Can you work these out from the model? Positions are in its coordinate system, mm. A direction names the side the tool comes from. Give positions to 0.01 mm unless a question says otherwise; leave off trailing zeros. Order: outer loops, then holes, each group sorted by start corner. A loop starts at its lowest first (then second) coordinate and runs counter-clockwise, first axis right, second up. Notation, with made-up numbers: M -32.75,54.5 L -19.75,54.5 A21 cw -19.75,83.5 Z; hole C -35,55.25 d3. An arc over 180 degrees is marked long. Write each question's results on one line, items separated by ' | '.
from build123d import *

# Parameters (mm, degrees)
F0_R     = 30
F0_R_2   = 20
F0_R_3   = 3.5
F1_DEPTH = 35
F2_DEPTH = 45
F3_DEPTH = 65
F6_DEPTH = 10
F7_R     = 3.5


with BuildPart() as f1:
    # F0 (on Top) → F1 (new body)
    with BuildSketch(Plane.XY):
        Circle(F0_R)
        Circle(F0_R_2, mode=Mode.SUBTRACT)
        Circle(F0_R_2)
        Circle(F0_R_3, mode=Mode.SUBTRACT)
    extrude(amount=-F1_DEPTH)

    # F0 (on Top) → F2 (join)
    with BuildSketch(Plane.XY):
        Circle(F0_R_2)
        Circle(F0_R_3, mode=Mode.SUBTRACT)
    extrude(amount=F2_DEPTH)

    # F0 (on Top) → F3 (join)
    with BuildSketch(Plane.XY):
        Circle(F0_R_3)
    extrude(amount=F3_DEPTH)

    # F5 (on offset) → F6 (join)
    with BuildSketch(Plane.XY.offset(65)):
        with BuildLine():
            Line((0, 3.582485), (0, 15))
            ThreePointArc((0, 15), (-10.606602, 10.606602), (-15, 0))
            Line((-15, 0), (-1.836112, 0))
            Line((-1.836112, 0), (-0.225955, 0))
            Line((-0.225955, 0), (0, -0.090901))
            Line((0, -0.090901), (0, -1.836112))
            Line((0, -1.836112), (0, -15))
            ThreePointArc((0, -15), (10.606602, -10.606602), (15, 0))
            Line((15, 0), (1.836112, 0))
            Line((1.836112, 0), (0.280118, 0))
            Line((0.280118, 0), (0, 0.357013))
            Line((0, 0.357013), (0, 3.582485))
        make_face()
    extrude(amount=F6_DEPTH)

    # F7
    f7_edges = [f1.edges().sort_by_distance(p)[0] for p in [
        (-20, 0, 45),
        (-30, 0, 0),
    ]]
    fillet(f7_edges, radius=F7_R)


solid = f1.part
(1) For faces 1 (the face through (7, -7, 65)), 2 (the face through (0, 8, 70)), 3 (the face through (-8, 0, 70)), 4 (the face through (3.233, -1.341, 54.86)), which set-ups out of +Z, -Z, +X, -X, +Y, -Y let a thin tool reach every point of the face, with its end or its side?
Data:
face 1: +X, -Y | face 2: +Z, +X, +Y | face 3: +Z, -X, -Y | face 4: none
(2) Will these pins go through, and if not, where does the flat tip stop? P1, Ø3, axis at x = 13.5, y = -22.5, coming from the +Z side; P2, Ø2, axis at x = -0.5, y = 0, coming from the -Z side; P3, Ø8, axis at x = -7, z = 71, coming from the -Y side; P4, Ø1.5, axis at y = -22, z = 16.5, coming from the +X side.
Data:
P1: stops at z = 0 | P2: stops at z = 0 | P3: stops at y = 0 | P4: passes through
(3) Imagine slicing it at A-A, the plane z = 37. Write out the boundary of the cut face in (x, y).
Data:
outline: C 0,0 d40
(4) We'd pull the mould along Y, two halves only. Please class faces 5 (the face through (3.233, -1.341, -17.745)), 6 (the face through (-10.49, 10.72, 69.93)), 7 (the face through (-4.336, -19.524, 20.46)), 8 (the face through (0, 0, 0)): +Y half, -Y half, draft (parallel to the pull), parting line (faces both ways), or undercut.
Data:
face 5: undercut | face 6: +Y half | face 7: parting line | face 8: undercut
(5) I need wall thicknesses on L1, parallel to Y at x = 0, z = -9; L2, parallel to Z at x = 11, y = -6; L3, parallel to Z at x = 24, y = -5. Which ranges of each line are inside material? Lowest first, please. Write a range as from..to.
Data:
L1: y = -30..-3.5, 3.5..30 | L2: z = -35..45, 65..75 | L3: z = -35..0
